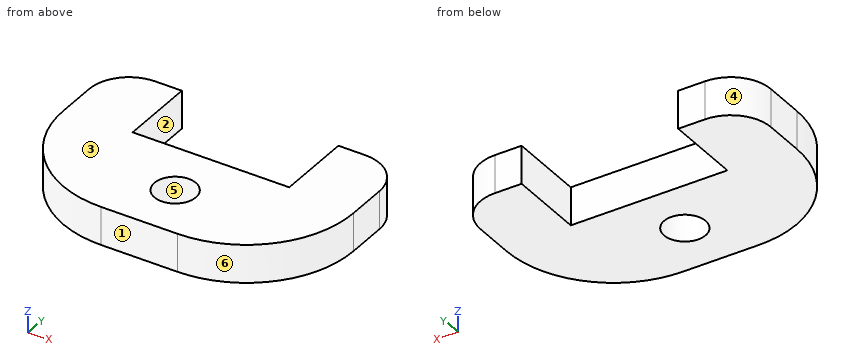
from build123d import *

# Parameters (mm, degrees)
BOSS_EXTRUDE1_DEPTH = 2.85
SKETCH2_R           = 1.55
CUT_EXTRUDE1_DEPTH  = 14.222896808
FILLET1_R           = 8
FILLET2_R           = 3


with BuildPart() as part:
    # Sketch1 → Boss-Extrude1 (new body)
    with BuildSketch(Plane.XY):
        Polygon((5.85, 7), (10.85, 7), (10.85, -7), (-10.85, -7), (-10.85, 7), (-5.85, 7), (-5.85, 1.3), (5.85, 1.3), align=None)
    extrude(amount=BOSS_EXTRUDE1_DEPTH)

    # Sketch2 → Cut-Extrude1 (cut, through all)
    with BuildSketch(Plane.XY.offset(2.85)):
        with Locations((0, -2.85)):
            Circle(SKETCH2_R)
    extrude(amount=-CUT_EXTRUDE1_DEPTH, mode=Mode.SUBTRACT)

    # Fillet1
    fillet1_edges = [part.edges().sort_by_distance(p)[0] for p in [
        (10.85, -7, 1.425),
        (-10.85, -7, 1.425),
    ]]
    fillet(fillet1_edges, radius=FILLET1_R)

    # Fillet2
    fillet2_edges = [part.edges().sort_by_distance(p)[0] for p in [
        (-10.85, 7, 1.425),
        (10.85, 7, 1.425),
    ]]
    fillet(fillet2_edges, radius=FILLET2_R)


solid = part.part
The listing builds one solid part. Answer for the finished solid, in the listing's coordinates (mm). Face numbers are marked on the shaded views. A direction names the side the tool comes from. Coordinates: 2 decimals unless noted, no trailing zeros. Write each loop counter-clockwise with the first axis right and the second up, starting at its lowest first coordinate (ties: lowest second). Pieces come first, ordered by that corner, then holes. Notation, with made-up numbers: M 70.25,25 L 80.25,25 A24 cw 80.25,37 Z; hole C 20,-7 d10. An arc over 180 degrees is marked long. Write each question's results on one line, items separated by ' | '.
Item 1: The part is cut by section B-B on x = 0. Determine the outline of the cut face in (y, z), and give its area (3 significant figures).
Answer below:
outline: M -7,0 L -4.4,0 L -4.4,2.85 L -7,2.85 Z; M -1.3,0 L 1.3,0 L 1.3,2.85 L -1.3,2.85 Z | area: 14.8 mm2
Item 2: The part is cut by section D-D on x = 6.5. Determine the outline of the cut face in (y, z).
Answer below:
outline: M -6.12,0 L 7,0 L 7,2.85 L -6.12,2.85 Z
Item 3: The part is cut by section A-A on y = 5.75. Determine the outline of the cut face in (x, z).
Answer below:
outline: M -10.29,0 L -5.85,0 L -5.85,2.85 L -10.29,2.85 Z; M 5.85,0 L 10.29,0 L 10.29,2.85 L 5.85,2.85 Z
Item 4: Given P1, Ø0.9, axis at y = 5.5, z = 1, coming from the +X side; P2, Ø8, axis at x = -2.5, y = -1, coming from the -Z side; P3, Ø1, axis at x = 6, z = 1, coming from the -Y side; P4, Ø1, axis at x = 8, z = 0.5, coming from the -Y side, each flat-ended and moving along its own axis, determine where each tip first touches the part or whether it passes through.
Answer below:
P1: x = 10.66 | P2: z = 0 | P3: y = -6.55 | P4: y = -5.51
Item 5: For a pull along X with two mould halves and no side action, classify the marked faces 3, 4, 5 and 6 as released by +X, released by -X, zero draft, split by the parting line, or undercut.
Answer below:
face 3: zero draft | face 4: released by -X | face 5: undercut | face 6: released by +X
Item 6: Consider probe 1 along X at (y, z) = (1.75, 0.15); probe 2 along Y at (x, z) = (0, 1.15). Determine where each line is inside the solid, lowest interval first. Write a range as [from, to].
Answer below:
probe 1: [-10.85, -5.85], [5.85, 10.85] | probe 2: [-7, -4.4], [-1.3, 1.3]
Item 7: Which of the six approach directions +Z, -Z, +X, -X, +Y, -Y give full straight-line access (tool end or side, diameter ignored) to the marked faces 1 and 2?
Answer below:
face 1: +Z, -Z, +X, -X, -Y | face 2: +Z, -Z, +Y
Item 8: The part is cut by section C-C on z = 1.3. Determine the outline of the cut face in (x, y), and give its area (3 significant figures).
Answer below:
outline: M -10.85,1 A8 ccw -2.85,-7 L 2.85,-7 A8 ccw 10.85,1 L 10.85,4 A3 ccw 7.85,7 L 5.85,7 L 5.85,1.3 L -5.85,1.3 L -5.85,7 L -7.85,7 A3 ccw -10.85,4 Z; hole C 0,-2.85 d3.1 | area: 198 mm2
